from build123d import *

# Parameters (mm, degrees)
SKETCH1_W            = 7.305999503
SKETCH1_H            = 15.829665589
BOSS_EXTRUDE1_DEPTH  = 250
SKETCH2_R            = 2.859737651
SKETCH2_R_2          = 3.043630703
SKETCH2_R_3          = 5.918472751
SKETCH2_R_4          = 4.573365308
CUT_EXTRUDE1_DEPTH   = 250
BOSS_EXTRUDE2_DEPTH  = 25
SKETCH4_R            = 0.55626985
SKETCH4_R_2          = 0.971483528
SKETCH4_R_3          = 0.995085758
SKETCH4_R_4          = 0.977672137
CUT_EXTRUDE2_DEPTH   = 2
SKETCH5_W            = 22.677292764
SKETCH5_H            = 18.650483769
BOSS_EXTRUDE3_DEPTH  = 10
SKETCH7_W            = 7.305999503
SKETCH7_H            = 15.829665589
BOSS_EXTRUDE4_DEPTH  = 15
SKETCH8_R            = 0.583511753
BOSS_EXTRUDE5_DEPTH  = 30
SKETCH10_R           = 1.176105539
SKETCH10_R_2         = 0.991111504
BOSS_EXTRUDE6_DEPTH  = 16.164956
SKETCH11_W           = 22.072449834
SKETCH11_H           = 15.598961577
SKETCH11_R           = 0.583511753
BOSS_EXTRUDE7_DEPTH  = 2
SKETCH12_W           = 8.462475972
SKETCH12_H           = 0.708060972
CUT_EXTRUDE3_DEPTH   = 16.949179392
SKETCH13_R           = 2.558098884
BOSS_EXTRUDE8_DEPTH  = 120
SKETCH14_W           = 4.036675172
SKETCH14_H           = 2.530453093
CUT_EXTRUDE4_DEPTH   = 3
SKETCH15_W           = 22.723161813
SKETCH15_H           = 26.77895865
BOSS_EXTRUDE9_DEPTH  = 3
SKETCH16_W           = 3.62280941
SKETCH16_H           = 0.845659338
BOSS_EXTRUDE10_DEPTH = 10
BOSS_EXTRUDE11_DEPTH = 3.622809
SKETCH20_W           = 9.26545532
SKETCH20_H           = 26.77895865
SKETCH20_R           = 2.555213065
SKETCH20_R_2         = 1.645957428
BOSS_EXTRUDE12_DEPTH = 3
FILLET1_R            = 3


with BuildPart() as part:
    # Sketch1 → Boss-Extrude1 (new body)
    with BuildSketch(Plane.XY):
        with Locations((3.652999752, 7.914832795)):
            Rectangle(SKETCH1_W, SKETCH1_H)
    extrude(amount=BOSS_EXTRUDE1_DEPTH)

    # Sketch2 → Cut-Extrude1 (cut)
    with BuildSketch(Plane(origin=(7.305999503, 0, 0), x_dir=(0, 0, -1), z_dir=(1, 0, 0))):
        with Locations((-228.573273141, 9.394450982)):
            Circle(SKETCH2_R)
        with Locations((-178.266254758, 9.394450982)):
            Circle(SKETCH2_R_2)
        with Locations((-85.722862653, 6.350820279)):
            Circle(SKETCH2_R_3)
        with Locations((-17.660426017, 6.350820279)):
            Circle(SKETCH2_R_4)
    extrude(amount=-CUT_EXTRUDE1_DEPTH, mode=Mode.SUBTRACT)

    # Sketch3 → Boss-Extrude2 (add)
    with BuildSketch(Plane.XY.offset(250)):
        Polygon((3.119708773, 18.218776332), (3.119708773, 15.829665589), (7.843143149, 15.829665589), (8.300249701, 0), (3.119708773, 0), (3.119708773, -2.731940657), (13.290329566, -2.731940657), (12.68534458, 18.218776332), align=None)
    extrude(amount=-BOSS_EXTRUDE2_DEPTH)

    # Sketch4 → Cut-Extrude2 (cut)
    with BuildSketch(Plane(origin=(13.200433203, 0.381183322, 0), x_dir=(0, 0, -1), z_dir=(0.999583332, 0.028864545, 0))):
        with Locations((-247.357123666, 16.004078596)):
            Circle(SKETCH4_R)
        with Locations((-228.271108715, 16.004078596)):
            Circle(SKETCH4_R_2)
        with Locations((-228.271108715, -0.707178735)):
            Circle(SKETCH4_R_3)
        with Locations((-246.800853817, -0.707178735)):
            Circle(SKETCH4_R_4)
    extrude(amount=-CUT_EXTRUDE2_DEPTH, mode=Mode.SUBTRACT)

    # Sketch5 → Boss-Extrude3 (add)
    with BuildSketch(Plane(origin=(13.200433203, 0.381183322, 0), x_dir=(0, 0, -1), z_dir=(0.999583332, 0.028864545, 0))):
        with Locations((-237.496397387, 7.284247631)):
            Rectangle(SKETCH5_W, SKETCH5_H)
    extrude(amount=BOSS_EXTRUDE3_DEPTH)

    # Sketch7 → Boss-Extrude4 (add)
    with BuildSketch(Plane.XY.offset(250)):
        with Locations((3.652999752, 7.914832795)):
            Rectangle(SKETCH7_W, SKETCH7_H)
    extrude(amount=BOSS_EXTRUDE4_DEPTH)

    # Sketch8 → Boss-Extrude5 (add)
    with BuildSketch(Plane.XY.offset(248.835043769)):
        with Locations((17.375180219, 7.845532394)):
            Circle(SKETCH8_R)
    extrude(amount=BOSS_EXTRUDE5_DEPTH)

    # Sketch10 → Boss-Extrude6 (add)
    with BuildSketch(Plane.XY.offset(248.835043769)):
        with Locations((17.375180219, 7.845532394)):
            Circle(SKETCH10_R)
        with Locations((17.375180219, 7.845532394)):
            Circle(SKETCH10_R_2, mode=Mode.SUBTRACT)
    extrude(amount=BOSS_EXTRUDE6_DEPTH)

    # Sketch11 → Boss-Extrude7 (add)
    with BuildSketch(Plane.XY.offset(265)):
        with Locations((11.036224917, 8.030184801)):
            Rectangle(SKETCH11_W, SKETCH11_H)
        with Locations((17.375180219, 7.845532394)):
            Circle(SKETCH11_R, mode=Mode.SUBTRACT)
    extrude(amount=BOSS_EXTRUDE7_DEPTH)

    # Sketch12 → Cut-Extrude3 (cut, through all)
    with BuildSketch(Plane(origin=(7.305999503, 0, 0), x_dir=(0, 0, -1), z_dir=(1, 0, 0))):
        with Locations((-257.232117953, 8.667607447)):
            Rectangle(SKETCH12_W, SKETCH12_H)
    extrude(amount=CUT_EXTRUDE3_DEPTH, mode=Mode.SUBTRACT)

    # Sketch13 → Boss-Extrude8 (add)
    with BuildSketch(Plane(origin=(23.196266525, 0.669828769, 0), x_dir=(0, 0, -1), z_dir=(0.999583332, 0.028864545, 0))):
        with Locations((-237.28625307, 6.924561564)):
            Circle(SKETCH13_R)
    extrude(amount=BOSS_EXTRUDE8_DEPTH)

    # Sketch14 → Cut-Extrude4 (cut)
    with BuildSketch(Plane(origin=(0.05891237, -2.040143836, 0), x_dir=(0.999583332, 0.028864545, 0), z_dir=(0.028864545, -0.999583332, 0))):
        with Locations((18.81578383, 228.781338254)):
            Rectangle(SKETCH14_W, SKETCH14_H)
    extrude(amount=-CUT_EXTRUDE4_DEPTH, mode=Mode.SUBTRACT)

    # Sketch15 → Boss-Extrude9 (add)
    with BuildSketch(Plane(origin=(0, 0, 0), x_dir=(-1, 0, 0), z_dir=(0, 0, -1))):
        with Locations((-11.361580907, 4.28062146)):
            Rectangle(SKETCH15_W, SKETCH15_H)
    extrude(amount=BOSS_EXTRUDE9_DEPTH)

    # Sketch16 → Boss-Extrude10 (add)
    with BuildSketch(Plane.XY):
        with Locations((17.811006308, -3.783209828)):
            Rectangle(SKETCH16_W, SKETCH16_H)
    extrude(amount=BOSS_EXTRUDE10_DEPTH)

    # Sketch17 → Boss-Extrude11 (add)
    with BuildSketch(Plane(origin=(19.622411013, 0, 0), x_dir=(0, 0, -1), z_dir=(1, 0, 0))):
        Polygon((-10, -3.360380159), (-9.219259529, -2.579639689), (-9.219259529, -3.360380159), align=None)
    extrude(amount=-BOSS_EXTRUDE11_DEPTH)

    # Sketch20 → Boss-Extrude12 (add)
    with BuildSketch(Plane.ZY):
        with Locations((-7.63272766, 4.28062146)):
            Rectangle(SKETCH20_W, SKETCH20_H)
        with Locations((-8.150644595, 12.915896002)):
            Circle(SKETCH20_R, mode=Mode.SUBTRACT)
        with Locations((-7.163070138, -4.86044422)):
            Circle(SKETCH20_R_2, mode=Mode.SUBTRACT)
    extrude(amount=-BOSS_EXTRUDE12_DEPTH)

    # Fillet1
    fillet1_edges = [part.edges().sort_by_distance(p)[0] for p in [
        (3, 4.28062146, -3),
    ]]
    fillet(fillet1_edges, radius=FILLET1_R)


solid = part.part
Source: CAD feature listing. Evaluate the final solid. Frame: model axes, mm. A direction names the side the tool comes from. Coordinates: 2 decimals unless noted, no trailing zeros. Order: outer loops, then holes, each group sorted by start corner. A loop starts at its lowest first (then second) coordinate and runs counter-clockwise, first axis right, second up.
Item 1: Cut plane B-B (z = 96.5). Return loops of the section in (x, y), plus the area to 3 significant figures.
Output values:
outline: (0, 0) - (7.31, 0) - (7.31, 15.83) - (0, 15.83) - close
area: 116 mm2
Item 2: Pull-direction query (Z, two-part tool) for faces 1 (the face through (82.11, 10.067, 234.846)), 2 (the face through (4, 0, 131)), 3 (the face through (1.48, 15.45, -8.48)), 4 (the face through (0, 7, 125)); classes: pulls with the +Z half, pulls with the -Z half, needs draft (parallel to the pull), parting line crosses it, or undercut.
Output values:
face 1: parting line crosses it
face 2: undercut
face 3: undercut
face 4: needs draft
Item 3: Cut plane A-A (z = 178). Return loops of the section in (x, y), plus the area to 3 significant figures.
Output values:
outline: (0, 0) - (7.31, 0) - (7.31, 6.36) - (0, 6.36) - close; (0, 12.43) - (7.31, 12.43) - (7.31, 15.83) - (0, 15.83) - close
area: 71.3 mm2
Item 4: First-contact query: P1, Ø8, axis at y = 12.92, z = -8.15, coming from the +X side; P2, Ø5.5, axis at x = 19.5, y = 9, coming from the -Z side; P3, Ø6, axis at y = 10, z = 117, coming from the +X side; P4, Ø6, axis at x = 107, y = 1.5, coming from the -Z side. Flat tips, straight axial feed; report the tip coordinate or a pass-through.
Output values:
P1: stops at x = 3.61
P2: stops at z = -3
P3: stops at x = 7.31
P4: passes through
Item 5: Set-up query: faces 5 (the face through (3.7, 9.52, 231.43)), 6 (the face through (8, 18.219, 238)). Return all of +Z, -Z, +X, -X, +Y, -Y with unobstructed straight access to the full face (end or side cutting, diameter ignored); none if empty.
Output values:
face 5: -X
face 6: +Z, -Z, +X, -X, +Y
Item 6: Material intervals for line 1 (Z direction, x = 18, y = 14.25); line 2 (X direction, y = 8.25, z = 257); line 3 (X direction, y = 5.25, z = 123), sorted ascending.
Output values:
line 1: z = -3 to 0, 226.16 to 248.84, 265 to 267
line 2: x = 0 to 7.31, 16.27 to 16.47, 16.95 to 17.8, 18.28 to 18.48
line 3: x = 0 to 7.31
